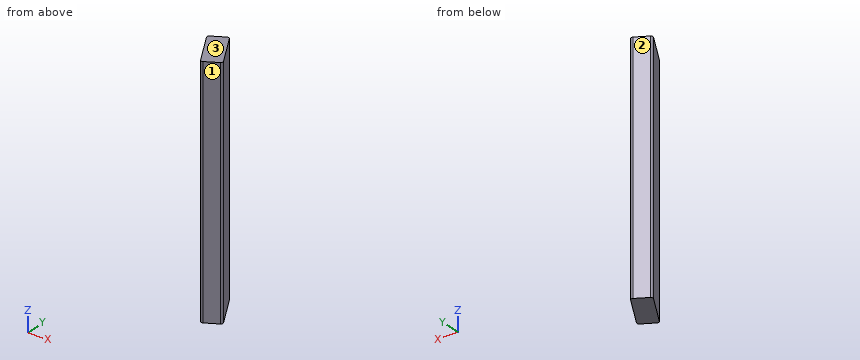
```python
from build123d import *

# Parameters (mm, degrees)
BOSS_EXTRUDE1_DEPTH = 490.537961
FILLET1_R           = 4.7625


with BuildPart() as part:
    # Sketch1 → Boss-Extrude1 (new body)
    with BuildSketch(Plane.XY):
        Polygon((227.693380197, -470.576503047), (183.243380197, -393.586844651), (216.238948081, -374.536844651), (260.688948081, -451.526503047), align=None)
    extrude(amount=BOSS_EXTRUDE1_DEPTH)

    # Fillet1
    fillet1_edges = [part.edges().sort_by_distance(p)[0] for p in [
        (227.693380197, -470.576503047, 245.2689805),
        (183.243380197, -393.586844651, 245.2689805),
        (216.238948081, -374.536844651, 245.2689805),
        (260.688948081, -451.526503047, 245.2689805),
    ]]
    fillet(fillet1_edges, radius=FILLET1_R)


solid = part.part
```
The model under review builds one solid part; all positions refer to its coordinate system, in mm. Face numbers are marked on the shaded views. Round coordinates to 2 decimals unless told otherwise and drop trailing zeros. Loops run counter-clockwise (first coordinate to the right, second up) from the corner with the lowest first, then second, coordinate; pieces in that order, holes last. Notation, with made-up numbers: M -18.75,17.25 L -11.75,17.25 A24 cw -11.75,42.25 Z; hole C 59,89 d8. An arc over 180 degrees is marked long. Write item = value, one per line.
Item 1: Take a section at B-B on x = 251. Write out the cut boundary in (y, z).
Return value:
outline = M -457.12,0 L -434.74,0 L -434.74,490.54 L -457.12,490.54 Z
Item 2: Take a section at A-A on z = 256. Write out the cut boundary in (x, y) (1 decimal), then the cut area to 3 significant figures.
Return value:
outline = M 185.6,-397.7 L 225.3,-466.5 A4.8 ccw 231.8,-468.2 L 256.6,-453.9 A4.8 ccw 258.3,-447.4 L 218.6,-378.7 A4.8 ccw 212.1,-376.9 L 187.4,-391.2 A4.8 ccw Z
area = 3,370 mm2
Item 3: The part is to be moulded in two halves that separate along Y. For the marked faces 1, 2 and 3, say which applies: released by +Y, released by -Y, zero draft, split by the parting line, or undercut.
Return value:
face_1 = released by -Y
face_2 = released by +Y
face_3 = zero draft
Item 4: Insertion check: P1, Ø10, axis at y = -395.5, z = 233.5, coming from the +X side; P2, Ø5, axis at y = -419.5, z = 306, coming from the -X side; P3, Ø3, axis at y = -425, z = 183, coming from the -X side; P4, Ø2, axis at x = 246, y = -456.5, coming from the -Z side. Each pin has a flat end and moves straight along its axis. Give the tip position at first contact, or say it passes through.
Return value:
P1 = 231.23
P2 = 196.76
P3 = 200.51
P4 = 0
Item 5: Take a section at C-C on y = -384. Write out the cut boundary in (x, z), then the cut area to 3 significant figures.
Return value:
outline = M 199.85,0 L 221.7,0 L 221.7,490.54 L 199.85,490.54 Z
area = 10,700 mm2
Item 6: For line 1 (Y direction, x = 240, z = 328); line 2 (Y direction, x = 234.5, z = 330); line 3 (X direction, y = -433.5, z = 443.5), list the stretches that pass through material, from the lowest coordinate up. Write a range as [from, to].
Return value:
line_1 = [-463.47, -415.69]
line_2 = [-466.65, -406.17]
line_3 = [206.29, 250.28]
